from build123d import *

# Parameters (mm, degrees)
SKETCH1_R           = 2.5
SKETCH1_R_2         = 4.1656
BOSS_EXTRUDE1_DEPTH = 3


with BuildPart() as part:
    # Sketch1 → Boss-Extrude1 (new body)
    with BuildSketch(Plane(origin=(0, 0, 0), x_dir=(1, 0, 0), z_dir=(0, 1, 0))):
        with BuildLine():
            Line((-108.6375, -53.522608696), (-108.6375, -86.542608696))
            ThreePointArc((-108.6375, -86.542608696), (-107.893551224, -88.33865992), (-106.0975, -89.082608696))
            Line((-106.0975, -89.082608696), (-24.8175, -89.082608696))
            ThreePointArc((-24.8175, -89.082608696), (-23.021448776, -88.33865992), (-22.2775, -86.542608696))
            Line((-22.2775, -86.542608696), (-22.2775, 86.177391304))
            ThreePointArc((-22.2775, 86.177391304), (-23.021448776, 87.973442529), (-24.8175, 88.717391304))
            Line((-24.8175, 88.717391304), (-106.0975, 88.717391304))
            ThreePointArc((-106.0975, 88.717391304), (-107.893551224, 87.973442529), (-108.6375, 86.177391304))
            Line((-108.6375, 86.177391304), (-108.6375, -10.342608696))
            ThreePointArc((-108.6375, -10.342608696), (-109.381448776, -12.13865992), (-111.1775, -12.882608696))
            Line((-111.1775, -12.882608696), (-182.2975, -12.882608696))
            ThreePointArc((-182.2975, -12.882608696), (-184.093551224, -13.626557471), (-184.8375, -15.422608696))
            Line((-184.8375, -15.422608696), (-184.8375, -48.442608696))
            ThreePointArc((-184.8375, -48.442608696), (-184.093551224, -50.23865992), (-182.2975, -50.982608696))
            Line((-182.2975, -50.982608696), (-111.1775, -50.982608696))
            ThreePointArc((-111.1775, -50.982608696), (-109.381448776, -51.726557471), (-108.6375, -53.522608696))
        make_face()
        with Locations(Location((-66.5475, 82.117391304, 0), (0, 0, 270))):
            Circle(SKETCH1_R, mode=Mode.SUBTRACT)
        with Locations(Location((-26.8975, 82.117391304, 0), (0, 0, 270))):
            Circle(SKETCH1_R, mode=Mode.SUBTRACT)
        with Locations(Location((-66.5475, 44.017391304, 0), (0, 0, 270))):
            Circle(SKETCH1_R, mode=Mode.SUBTRACT)
        with Locations(Location((-26.8975, 44.017391304, 0), (0, 0, 270))):
            Circle(SKETCH1_R, mode=Mode.SUBTRACT)
        with Locations(Location((-26.8975, -44.382608696, 0), (0, 0, 90))):
            Circle(SKETCH1_R, mode=Mode.SUBTRACT)
        with Locations(Location((-66.5475, -44.382608696, 0), (0, 0, 90))):
            Circle(SKETCH1_R, mode=Mode.SUBTRACT)
        with Locations(Location((-26.8975, -82.482608696, 0), (0, 0, 90))):
            Circle(SKETCH1_R, mode=Mode.SUBTRACT)
        with Locations(Location((-66.5475, -82.482608696, 0), (0, 0, 90))):
            Circle(SKETCH1_R, mode=Mode.SUBTRACT)
        with Locations(Location((-89.5875, -70.032608696, 0), (0, 0, 270))):
            Circle(SKETCH1_R_2, mode=Mode.SUBTRACT)
        with Locations(Location((-89.5875, 6.167391304, 0), (0, 0, 270))):
            Circle(SKETCH1_R_2, mode=Mode.SUBTRACT)
        with Locations(Location((-89.5875, 56.967391304, 0), (0, 0, 270))):
            Circle(SKETCH1_R_2, mode=Mode.SUBTRACT)
        with Locations(Location((-172.1375, -31.932608696, 0), (0, 0, 270))):
            Circle(SKETCH1_R_2, mode=Mode.SUBTRACT)
        with Locations(Location((-146.7375, -31.932608696, 0), (0, 0, 270))):
            Circle(SKETCH1_R_2, mode=Mode.SUBTRACT)
    extrude(amount=BOSS_EXTRUDE1_DEPTH)


solid = part.part
The model under review builds one solid part; all positions refer to its coordinate system, in mm. Round coordinates to 2 decimals unless told otherwise and drop trailing zeros. Order: outer loops, then holes, each group sorted by start corner. A loop starts at its lowest first (then second) coordinate and runs counter-clockwise, first axis right, second up. Notation, with made-up numbers: (-12, 41.5) -> (17, 41.5) arc R26 cw to (17, 68.5) -> close; hole circle Ø6 at (7.5, 50). An arc over 180 degrees is marked (long way). Return JSON: item names as keys, results as strings.
1. Take a section at D-D (z = 32.5). Write out the cut boundary in (x, y), then the cut area to 3 significant figures.
Answer block:
{"outline": "(-184.84, 0) -> (-176.26, 0) -> (-176.26, 3) -> (-184.84, 3) -> close; (-168.01, 0) -> (-150.86, 0) -> (-150.86, 3) -> (-168.01, 3) -> close; (-142.61, 0) -> (-22.28, 0) -> (-22.28, 3) -> (-142.61, 3) -> close", "area": "438 mm²"}
2. Take a section at B-B (z = -44). Write out the cut boundary in (x, y), then the cut area to 3 significant figures.
Answer block:
{"outline": "(-108.64, 0) -> (-69.05, 0) -> (-69.05, 3) -> (-108.64, 3) -> close; (-64.05, 0) -> (-29.4, 0) -> (-29.4, 3) -> (-64.05, 3) -> close; (-24.4, 0) -> (-22.28, 0) -> (-22.28, 3) -> (-24.4, 3) -> close", "area": "229 mm²"}
3. The part is to be moulded in two halves that separate along Z. For faces 1 (the face through (-27.01, 1.48, 84.98)), 2 (the face through (-87, 3, -1)), say which applies: +Z half, -Z half, draft (parallel to the pull), parting line (faces both ways), or undercut.
Answer block:
{"face 1": "undercut", "face 2": "draft"}
4. Take a section at A-A (y = 1). State how many separate pieces and enclosed holes the cut face has, then the cut area to 3 significant figures.
Answer block:
{"separate pieces": "1", "enclosed holes": "13", "area": "17,800 mm²"}
5. Take a section at C-C (z = 71). Write out the cut boundary in (x, y), then the cut area to 3 significant figures.
Answer block:
{"outline": "(-108.64, 0) -> (-93.64, 0) -> (-93.64, 3) -> (-108.64, 3) -> close; (-85.54, 0) -> (-22.28, 0) -> (-22.28, 3) -> (-85.54, 3) -> close", "area": "235 mm²"}
6. Insertion check: P1, Ø7.5, axis at x = -89.59, z = -56.97, coming from the -Y side. The pin has a flat end and moves straight along its axis. Give the tip position at first contact, or say it passes through.
Answer block:
{"P1": "passes through"}
7. For L1, parallel to Z at x = -147, y = 0.45; L2, parallel to Z at x = -92, y = 0.35; L3, parallel to Z at x = -177.5, y = 2.65, list the stretches that pass through material, from the lowest coordinate up. Write a range as [from, to].
Answer block:
{"L1": "z = [12.88, 27.78], [36.09, 50.98]", "L2": "z = [-88.72, -60.36], [-53.57, -9.56], [-2.77, 66.64], [73.43, 89.08]", "L3": "z = [12.88, 50.98]"}
